Source: CAD feature listing. Evaluate the final solid. Frame: model axes, mm. Face numbers are marked on the shaded views. Round coordinates to 2 decimals unless told otherwise and drop trailing zeros. Order: outer loops, then holes, each group sorted by start corner. A loop starts at its lowest first (then second) coordinate and runs counter-clockwise, first axis right, second up. Notation, with made-up numbers: (74, 48.5) -> (100, 48.5) arc R15 ccw to (100, 60.5) -> close; hole circle Ø5 at (62, -34). An arc over 180 degrees is marked (long way). One line per item, written item: value. Start each with the question number.
1) Section A-A (x = 0). Return the cut outline in (y, z) (3 decimals), and give its area (3 significant figures).
2) Pin query (flat end, axial travel): P1, Ø2, axis at y = 67, z = 24, coming from the -X side; P2, Ø5, axis at x = -22.5, y = 53.5, coming from the +Z side; P3, Ø5, axis at x = -83.5, y = 80.5, coming from the -Z side; P4, Ø8, axis at x = 53, z = -27, coming from the +Y side. Return the tip coordinate at first contact, or that it passes through.
3) Section C-C (z = 0). Return the cut outline in (x, y) (3 decimals).
4) Mould query, pull axis Z, two halves, no side actions, for the marked faces 1, 2 and 3. Classes: pulls with the +Z half, pulls with the -Z half, needs draft (parallel to the pull), parting line crosses it, or undercut.
5) Ray query, L1, parallel to X at y = 72.5, z = -7; L2, parallel to X at y = 33, z = 43; L3, parallel to Y at x = 66.5, z = 14. Return the intervals inside material, ascending.
6) Section D-D (x = -69). Return the cut outline in (y, z), and give its area (3 significant figures).
7) Section B-B (z = -49). Return the cut outline in (x, y) (3 decimals).
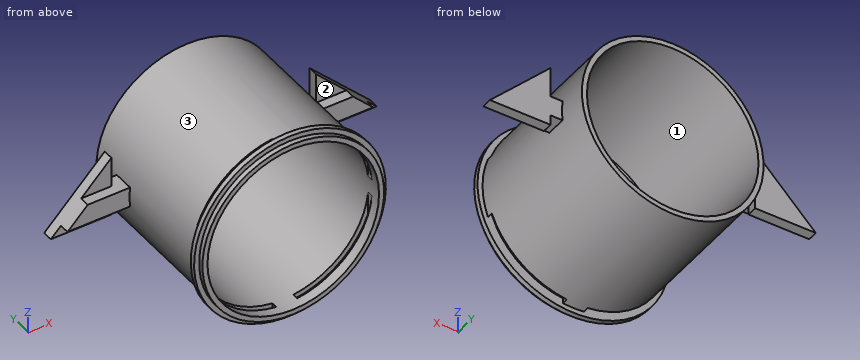
```python
from build123d import *

# Parameters (mm, degrees)
SKETCH1_R               = 57.15
BOSS_EXTRUDE1_DEPTH     = 101.6
SKETCH2_R               = 53.975
CUT_EXTRUDE1_DEPTH      = 130.826056707
CUT_EXTRUDE4_DEPTH      = 130.826056707
CUT_EXTRUDE4_DEPTH_BACK = 130.826056707
SKETCH6_W               = 47.117
SKETCH6_H               = 3.683
BOSS_EXTRUDE7_START     = 3.175
SKETCH10_R              = 60.325
SKETCH10_R_2            = 57.15
BOSS_EXTRUDE7_DEPTH     = 3.175
BOSS_EXTRUDE6_START     = 12.7
BOSS_EXTRUDE6_DEPTH     = 12.7
BOSS_EXTRUDE8_DEPTH     = 6.35


with BuildPart() as part:
    # Sketch1 → Boss-Extrude1 (new body)
    with BuildSketch(Plane(origin=(0, 0, 0), x_dir=(1, 0, 0), z_dir=(0, 1, 0))):
        with Locations(Location((0, 0, 0), (0, 0, 270))):
            Circle(SKETCH1_R)
    extrude(amount=BOSS_EXTRUDE1_DEPTH)

    # Sketch2 → Cut-Extrude1 (cut, through all)
    with BuildSketch(Plane(origin=(0, 101.6, 0), x_dir=(1, 0, 0), z_dir=(0, 1, 0))):
        with Locations(Location((0, 0, 0), (0, 0, 270))):
            Circle(SKETCH2_R)
    extrude(amount=-CUT_EXTRUDE1_DEPTH, mode=Mode.SUBTRACT)

    # Sketch6 → Cut-Extrude4 (cut, two sides: drawn at the far end of the back side and taken through both)
    with BuildSketch(Plane.XY.offset(-CUT_EXTRUDE4_DEPTH_BACK)):
        with Locations((-30.1625, 8.1915)):
            Rectangle(SKETCH6_W, SKETCH6_H)
        with Locations((30.1625, 8.1915)):
            Rectangle(SKETCH6_W, SKETCH6_H)
    extrude(amount=CUT_EXTRUDE4_DEPTH + CUT_EXTRUDE4_DEPTH_BACK, mode=Mode.SUBTRACT)

    # Sketch10 → Boss-Extrude7 (add)
    with BuildSketch(Plane(origin=(0, 0, 0), x_dir=(1, 0, 0), z_dir=(0, 1, 0)).offset(BOSS_EXTRUDE7_START)):
        with Locations(Location((0, 0, 0), (0, 0, 270))):
            Circle(SKETCH10_R)
        with Locations(Location((0, 0, 0), (0, 0, 270))):
            Circle(SKETCH10_R_2, mode=Mode.SUBTRACT)
    extrude(amount=BOSS_EXTRUDE7_DEPTH)

    # Sketch9 → Boss-Extrude6 (add)
    with BuildSketch(Plane(origin=(0, 69.85, 0), x_dir=(1, 0, 0), z_dir=(0, 1, 0)).offset(BOSS_EXTRUDE6_START)):
        with BuildLine():
            Line((-83.4525636, -6.35), (-53.600169076, -6.35))
            ThreePointArc((-53.600169076, -6.35), (-53.975, 0), (-53.600169076, 6.35))
            Line((-53.600169076, 6.35), (-96.1525636, 6.35))
            Line((-96.1525636, 6.35), (-83.4525636, -6.35))
        make_face()
    boss_extrude6 = extrude(amount=-BOSS_EXTRUDE6_DEPTH)

    # Sketch11 → Boss-Extrude8 (add)
    with BuildSketch(Plane(origin=(0, 82.55, 0), x_dir=(1, 0, 0), z_dir=(0, 1, 0))):
        Polygon((-64.4025636, -25.4), (-64.4025636, 12.7), (-102.5025636, 12.7), align=None)
    boss_extrude8 = extrude(amount=-BOSS_EXTRUDE8_DEPTH)

    # Mirror1: Boss-Extrude6, Boss-Extrude8 across plane
    add(boss_extrude6.mirror(Plane(origin=(0, 0, 0), x_dir=(0, 0, 1), z_dir=(1, 0, 0))))
    add(boss_extrude8.mirror(Plane(origin=(0, 0, 0), x_dir=(0, 0, 1), z_dir=(1, 0, 0))))


solid = part.part
```
Findings:
1. outline: (0, -57.15) -> (3.175, -57.15) -> (3.175, -60.325) -> (6.35, -60.325) -> (6.35, -57.15) -> (101.6, -57.15) -> (101.6, -53.975) -> (0, -53.975) -> close; (0, 53.975) -> (101.6, 53.975) -> (101.6, 57.15) -> (6.35, 57.15) -> (6.35, 60.325) -> (3.175, 60.325) -> (3.175, 57.15) -> (0, 57.15) -> close
1. area: 665 mm2
2. P1: x = -52.32
2. P2: z = 53.54
2. P3: z = -12.7
2. P4: y = 101.6
3. outline: (-89.803, 69.85) -> (-57.15, 69.85) -> (-57.15, 6.35) -> (-60.325, 6.35) -> (-60.325, 3.175) -> (-57.15, 3.175) -> (-57.15, 0) -> (-53.975, 0) -> (-53.975, 101.6) -> (-57.15, 101.6) -> (-57.15, 82.55) -> (-89.803, 82.55) -> close; (53.975, 0) -> (57.15, 0) -> (57.15, 3.175) -> (60.325, 3.175) -> (60.325, 6.35) -> (57.15, 6.35) -> (57.15, 69.85) -> (89.803, 69.85) -> (89.803, 82.55) -> (57.15, 82.55) -> (57.15, 101.6) -> (53.975, 101.6) -> close
4. face 1: undercut
4. face 2: needs draft
4. face 3: parting line crosses it
5. L1: -56.72 to -53.52, 53.52 to 56.72
5. L2: -37.64 to -32.62, 32.62 to 37.64
5. L3: 76.2 to 82.55
6. outline: (69.85, -6.35) -> (76.2, -6.35) -> (76.2, -12.7) -> (82.55, -12.7) -> (82.55, 20.8) -> (76.2, 20.8) -> (76.2, 6.35) -> (69.85, 6.35) -> close
6. area: 293 mm2
7. outline: (-35.187, 3.175) -> (-29.413, 3.175) -> (-29.413, 0) -> (-22.634, 0) -> (-22.634, 6.35) -> (-35.187, 6.35) -> close; (-29.413, 10.033) -> (-22.634, 10.033) -> (-22.634, 101.6) -> (-29.413, 101.6) -> close; (22.634, 0) -> (29.413, 0) -> (29.413, 3.175) -> (35.187, 3.175) -> (35.187, 6.35) -> (22.634, 6.35) -> close; (22.634, 10.033) -> (29.413, 10.033) -> (29.413, 101.6) -> (22.634, 101.6) -> close
